Geometry: see drawing. Coordinates: mm, zero at the bounding-box minimum. A direction names the side the tool comes from. Coordinates: 2 decimals unless noted, no trailing zeros. Order: outer loops, then holes, each group sorted by start corner. A loop starts at its lowest first (then second) coordinate and runs counter-clockwise, first axis right, second up. Notation, with made-up numbers: M -24.5,-31.75 L 22.5,-31.75 A24 cw 22.5,-8.75 Z; hole C -30,59.25 d5. An arc over 180 degrees is marked long. One line per item, written item: value.
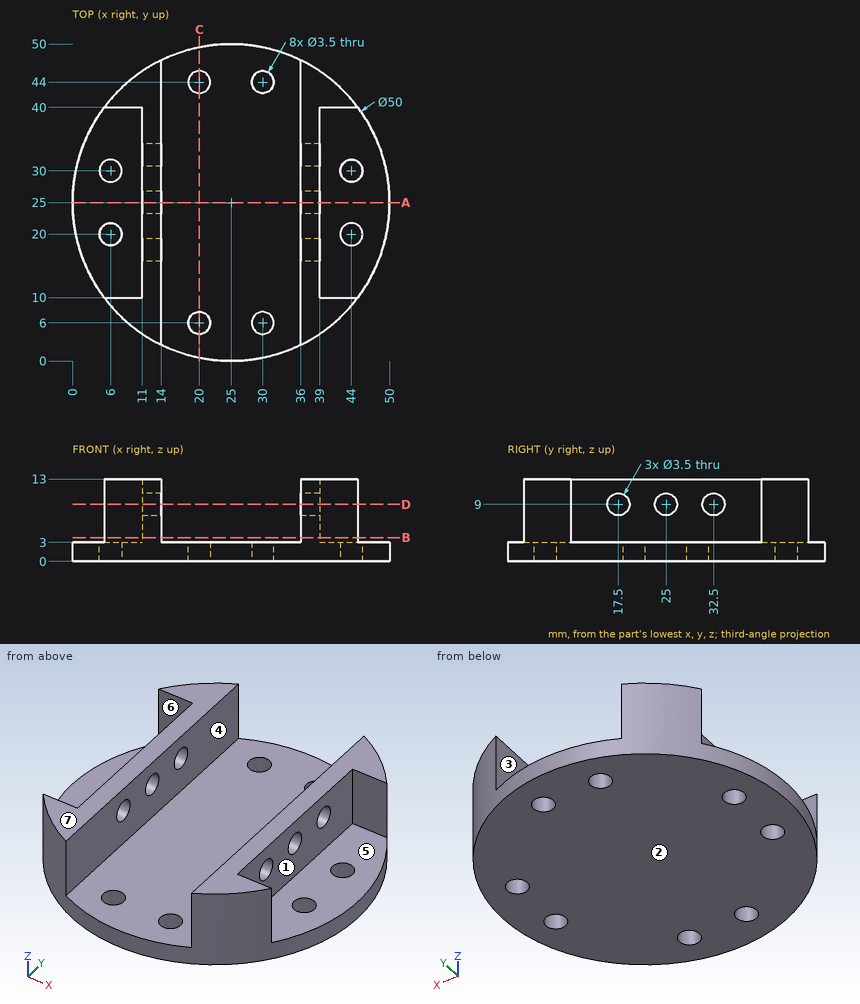
(1) Draft query along X for the marked faces 1, 2 and 3. Return one class per face: released by +X, released by -X, zero draft, split by the parting line, or undercut.
Data:
face 1: released by +X
face 2: zero draft
face 3: undercut
(2) Ray query, line 1 (Y direction, x = 30, z = 1.6); line 2 (X direction, y = 18.5, z = 3.5); line 3 (Y direction, x = 11.6, z = 9). Return the intervals inside material, ascending. Write a range as from..to.
Data:
line 1: y = 0.51..4.25, 7.75..42.25, 45.75..49.49
line 2: x = 11..14, 36..39
line 3: y = 3.89..15.75, 19.25..23.25, 26.75..30.75, 34.25..46.11
(3) Cut plane C-C on x = 20. Output: boundary loops of the cut face in (y, z), plus the area to 3 significant figures.
Data:
outline: M 0.51,0 L 4.25,0 L 4.25,3 L 0.51,3 Z; M 7.75,0 L 42.25,0 L 42.25,3 L 7.75,3 Z; M 45.75,0 L 49.49,0 L 49.49,3 L 45.75,3 Z
area: 126 mm2
(4) Cut plane A-A on y = 25. Output: boundary loops of the cut face in (x, z).
Data:
outline: M 0,0 L 50,0 L 50,3 L 39,3 L 39,7.25 L 36,7.25 L 36,3 L 14,3 L 14,7.25 L 11,7.25 L 11,3 L 0,3 Z; M 11,10.75 L 14,10.75 L 14,13 L 11,13 Z; M 36,10.75 L 39,10.75 L 39,13 L 36,13 Z
(5) Access query for the marked faces 4, 5, 6 and 7. Directions: +Z, -Z, +X, -X, +Y, -Y. A direction counts if a zero-diameter tool reaches every point of the face in a straight line with its end or side. Return the directions, or none.
Data:
face 4: +Z, +Y, -Y
face 5: +Z, +X
face 6: +Z, -X
face 7: +Z, +X, -X, +Y, -Y
(6) Cut plane D-D on z = 9. Give the number of separate pieces and of enclosed holes in the cut face, plus the area to 3 significant figures.
Data:
separate pieces: 8
enclosed holes: 0
area: 273 mm2
(7) Cut plane B-B on z = 3.75. Output: boundary loops of the cut face in (x, y), plus the area to 3 significant figures.
Data:
outline: M 5,10 A25 ccw 14,2.55 L 14,47.45 A25 ccw 5,40 L 11,40 L 11,10 Z; M 36,2.55 A25 ccw 45,10 L 39,10 L 39,40 L 45,40 A25 ccw 36,47.45 Z
area: 336 mm2
(8) First-contact query: pin 1 (4 mm diameter, centred on y = 21, z = 10.5, fed in from +X); pin 2 (12 mm diameter, centred on x = 46, y = 21.5, fed in from +Z); pin 3 (3 mm diameter, centred on y = 36, z = 1.5, fed in from -X). Flat tips, straight axial feed; report the tip coordinate or a pass-through.
Data:
pin 1: stops at x = 39
pin 2: stops at z = 3
pin 3: stops at x = 1.88
